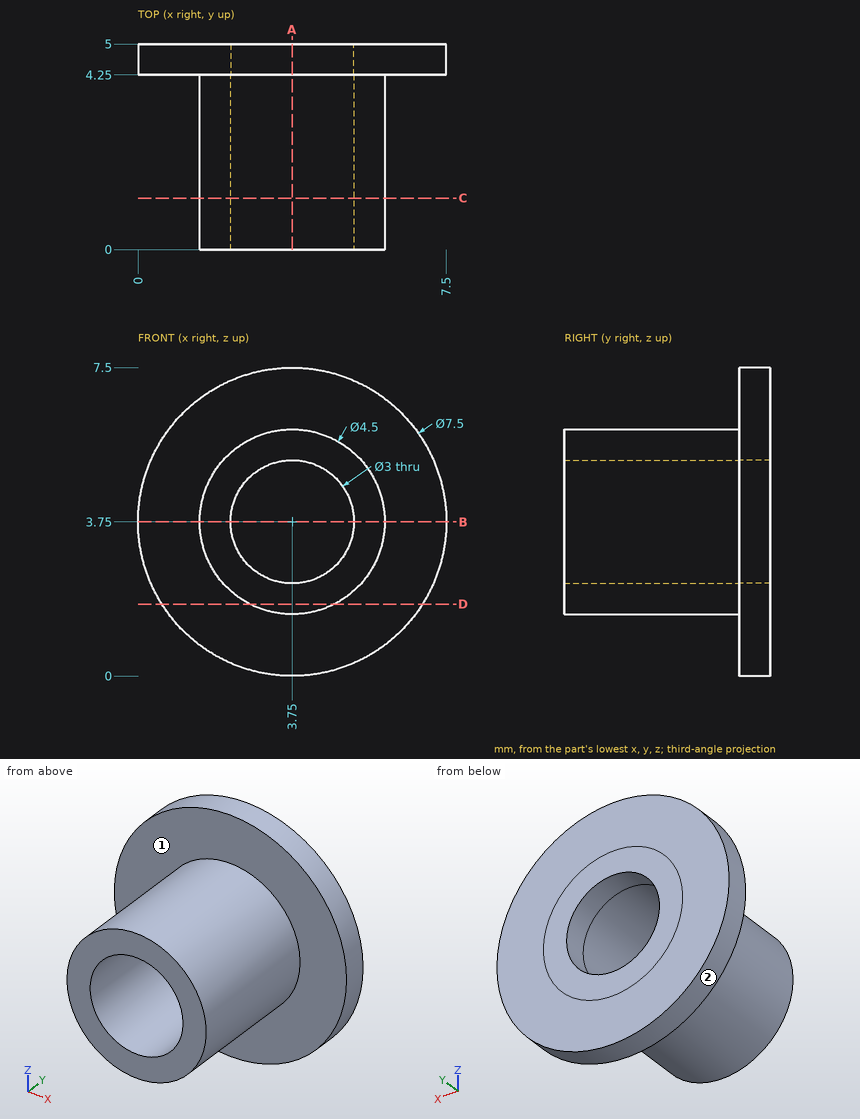
Geometry: see drawing. Coordinates: mm, zero at the bounding-box minimum. A direction names the side the tool comes from. Give positions to 0.01 mm unless a question says otherwise; leave off trailing zeros. Write each loop counter-clockwise with the first axis right and the second up, starting at its lowest first coordinate (ties: lowest second). Pieces come first, ordered by that corner, then holes. Notation, with made-up numbers: (14, 62.5) - (58, 62.5) arc R16 ccw to (58, 69.5) - close; hole circle Ø8 at (-29, 44.5). An arc over 180 degrees is marked (long way). Return JSON: item names as keys, results as strings. Group by question number.
1) Set-up query: the marked faces 1 and 2. Return all of +Z, -Z, +X, -X, +Y, -Y with unobstructed straight access to the full face (end or side cutting, diameter ignored); none if empty.
2) Line query: line 1 (X direction, y = 0.6, z = 3.75); line 2 (Z direction, x = 3.75, y = 4.6). Output: solid intervals per line, ascending.
3) Section A-A on x = 3.75. Return the cut outline in (y, z), plus the area to 3 significant figures.
4) Section B-B on z = 3.75. Return the cut outline in (x, y).
5) First-contact query: P1, Ø1.8, axis at x = 3.75, z = 3.75, coming from the -Y side; P2, Ø1.5, axis at x = 5.5, z = 1, coming from the -Y side; P3, Ø3, axis at y = 2.5, z = 1, coming from the +X side; P4, Ø3, axis at x = 2, y = 3, coming from the +Z side. Flat tips, straight axial feed; report the tip coordinate or a pass-through.
6) Section D-D on z = 1.75. Return the cut outline in (x, y).
7) Section C-C on y = 1.25. Return the cut outline in (x, z).
Filled in:
{
 "1": {"face 1": "-Y", "face 2": "+Y, -Y"},
 "2": {"line 1": "x = 1.5 to 2.25, 5.25 to 6", "line 2": "z = 0 to 2.25, 5.25 to 7.5"},
 "3": {"outline": "(0, 1.5) - (4.25, 1.5) - (4.25, 0) - (5, 0) - (5, 2.25) - (0, 2.25) - close; (0, 5.25) - (5, 5.25) - (5, 7.5) - (4.25, 7.5) - (4.25, 6) - (0, 6) - close", "area": "9.75 mm^2"},
 "4": {"outline": "(0, 4.25) - (1.5, 4.25) - (1.5, 0) - (2.25, 0) - (2.25, 5) - (0, 5) - close; (5.25, 0) - (6, 0) - (6, 4.25) - (7.5, 4.25) - (7.5, 5) - (5.25, 5) - close"},
 "5": {"P1": "passes through", "P2": "stops at y = 4.25", "P3": "stops at x = 5.62", "P4": "stops at z = 7.39"},
 "6": {"outline": "(0.58, 4.25) - (2.72, 4.25) - (2.72, 0) - (4.78, 0) - (4.78, 4.25) - (6.92, 4.25) - (6.92, 5) - (0.58, 5) - close"},
 "7": {"outline": "circle Ø4.5 at (3.75, 3.75); hole circle Ø3 at (3.75, 3.75)"}
}
